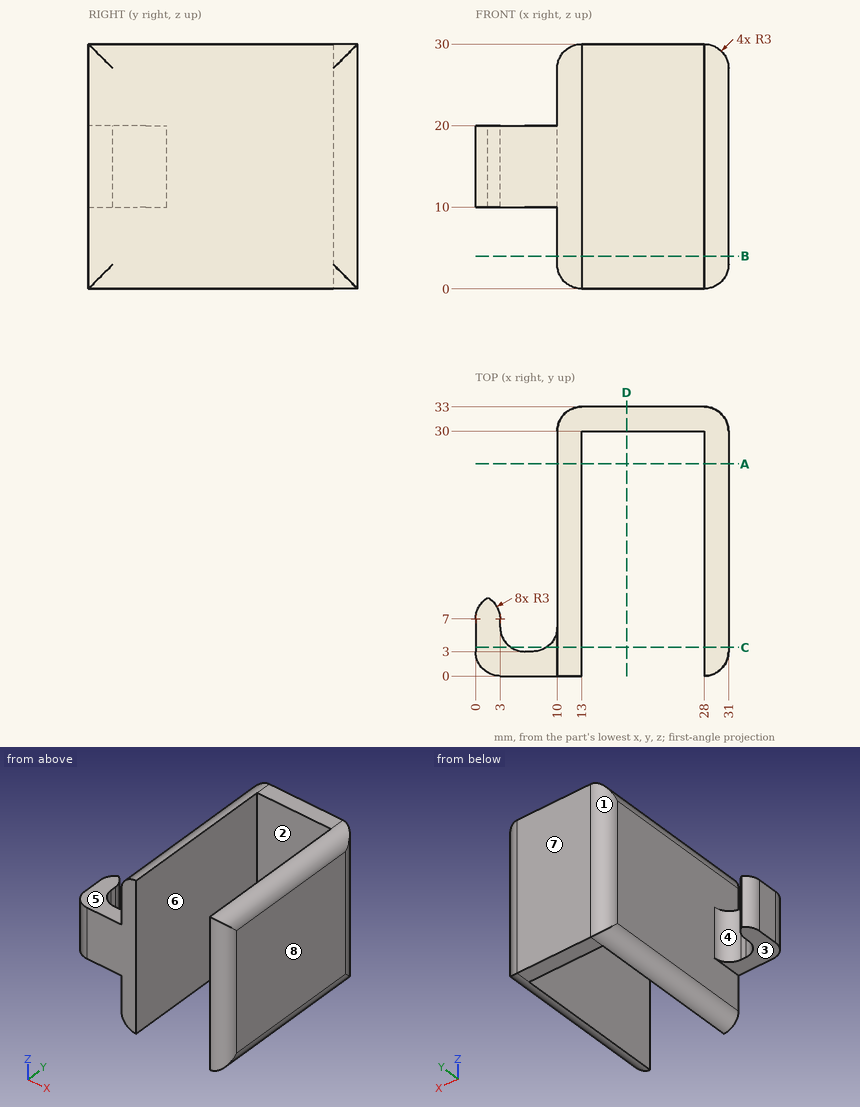
Verification items for this drawing (mm, ordinates from the low corner). A direction names the side the tool comes from. Coordinates: 2 decimals unless noted, no trailing zeros. Loops run counter-clockwise (first coordinate to the right, second up) from the corner with the lowest first, then second, coordinate; pieces in that order, holes last. Notation, with made-up numbers: (-17, 4) - (-7, 4) arc R22 ccw to (-7, 15) - close; hole circle Ø2 at (45, 58). An arc over 180 degrees is marked (long way). Use one line per item in the form item = value. Start each with the question number.
Item 1: Gauge pin test, flat ends, axial feed: pin 1 (0.8 mm diameter, centred on x = 6.5, z = 17, fed in from +Y); pin 2 (8 mm diameter, centred on y = 24.5, z = 20, fed in from -X); pin 3 (5 mm diameter, centred on x = 2.5, y = 6, fed in from -Z). Record the tip position at first contact, or that the pin passes through.
Item 2: Mould release check, pull along X, two halves, no side actions. Record for the marked faces 6, 7 and 8: +X half, -X half, draft (parallel to the pull), parting line (faces both ways), or undercut.
Item 3: Section check B-B, the plane z = 4. Enter the section's corners in (x, y), and give its area (3 significant figures).
Item 4: Section check A-A, the plane y = 26. Enter the section's corners in (x, z).
Item 5: Thickness scan on probe 1 along X at (y, z) = (6.5, 19.5); probe 2 along X at (y, z) = (12.5, 14.75); probe 3 along X at (y, z) = (4, 14.5). Record the ranges inside material, lowest first.
Item 6: Tool access check on the marked faces 1, 2, 3, 4 and 5. Record the directions out of +Z, -Z, +X, -X, +Y, -Y that give a thin tool (end or side, any length) a straight path to the whole face; none if there is none.
Item 7: Section check D-D, the plane x = 18.5. Enter the section's corners in (y, z), and give its area (3 significant figures).
Item 8: Section check C-C, the plane y = 3.5. Enter the section's corners in (x, z).
Computed:
q1.pin_1 = 3
q1.pin_2 = 10
q1.pin_3 = 10
q2.face_6 = undercut
q2.face_7 = draft
q2.face_8 = +X half
q3.outline = (10, 0) - (13, 0) - (13, 30) - (28, 30) - (28, 0) arc R3 ccw to (31, 3) - (31, 30) arc R3 ccw to (28, 33) - (13, 33) arc R3 ccw to (10, 30) - close
q3.area = 237 mm2
q4.outline = (10, 3) arc R3 ccw to (13, 0) - (13, 30) arc R3 ccw to (10, 27) - close; (28, 0) arc R3 ccw to (31, 3) - (31, 27) arc R3 ccw to (28, 30) - close
q5.probe_1 = 0 to 3, 10 to 13, 28 to 31
q5.probe_2 = 10 to 13, 28 to 31
q5.probe_3 = 0 to 3.76, 9.24 to 13, 28 to 31
q6.face_1 = +Z, -Z, -X, +Y
q6.face_2 = +Z, -Z, -Y
q6.face_3 = -Z, -X, +Y, -Y
q6.face_4 = +Z, -Z, +Y
q6.face_5 = +Z, -X, +Y, -Y
q7.outline = (30, 0) - (33, 0) - (33, 30) - (30, 30) - close
q7.area = 90.0 mm2
q8.outline = (0, 10) - (4.34, 10) - (4.34, 20) - (0, 20) - close; (8.66, 10) - (10, 10) - (10, 3) arc R3 ccw to (13, 0) - (13, 30) arc R3 ccw to (10, 27) - (10, 20) - (8.66, 20) - close; (28, 0) arc R3 ccw to (31, 3) - (31, 27) arc R3 ccw to (28, 30) - close
